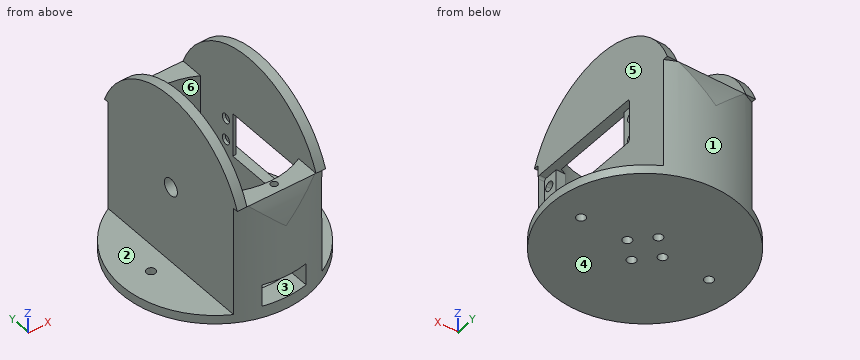
Autodesk Inventor part; units mm, degrees
ref_plane "РабПлоскость2" through (0, -42.5, 39) normal (0, -1, 0) x (1, 0, 0)
ref_plane "YZ Plane" through (0, 0, 0) normal (1, 0, 0) x (0, 1, 0)
ref_plane "XZ Plane" through (0, 0, 0) normal (0, 1, 0) x (-1, 0, 0)
sketch "Эскиз1" plane through (0, 0, 0) normal (0, 0, 1) x (1, 0, 0)
  circle A0 centre (29, 0) radius 2
  circle A1 centre (-29, 0) radius 2
  circle A2 centre (0, 8) radius 2
  circle A3 centre (8, 0) radius 2
  circle A4 centre (0, -8) radius 2
  circle A5 centre (-8, 0) radius 2
  circle A6 centre (0, 0) radius 42.5
  circle A7 centre (29, 0) radius 2
  circle A8 centre (-29, 0) radius 2
  circle A9 centre (0, 8) radius 2
  circle A10 centre (8, 0) radius 2
  circle A11 centre (0, -8) radius 2
  circle A12 centre (-8, 0) radius 2
  circle A13 centre (0, 0) radius 42.5
extrude "Выдавливание1" add sketch "Эскиз1" along normal blind 4
sketch "Эскиз16" plane through (0, 0, 4) normal (0, 0, 1) x (1, 0, 0)
  line L0 (-20, -37.5) -> (-20, 37.5)
  line L1 (20, 37.5) -> (20, -37.5)
  line L2 (20, -42.5) -> (-20, 42.5) construction
  line L3 (-20, -42.5) -> (20, 42.5) construction
  circle A0 centre (0, 0) radius 42.5
  arc A1 (-20, -37.5) -> (20, -37.5) centre (0, 0) ccw
  arc A2 (20, 37.5) -> (-20, 37.5) centre (0, 0) ccw
extrude "Выдавливание14" add sketch "Эскиз16" along normal blind 50 contours L0 A0 L1
sketch "Эскиз17" plane through (0, 0, 54) normal (0, 0, 1) x (1, 0, 0)
  line L0 (-15.66, -29.3625) -> (-15.66, 29.3625)
  line L1 (15.66, 29.3625) -> (15.66, -29.3625)
  line L2 (15.66, -33.2775) -> (-15.66, 33.2775) construction
  line L3 (-15.66, -33.2775) -> (15.66, 33.2775) construction
  arc A0 (-15.66, -29.3625) -> (15.66, -29.3625) centre (0, 0) ccw
  arc A1 (15.66, 29.3625) -> (-15.66, 29.3625) centre (0, 0) ccw
  arc A2 (-15.66, -29.3625) -> (15.66, -29.3625) centre (0, 0) ccw
  arc A3 (15.66, 29.3625) -> (-15.66, 29.3625) centre (0, 0) ccw
extrude "Выдавливание15" cut sketch "Эскиз17" against normal up to surface (50 mm away)
sketch "Эскиз23" plane through (-20, -37.5, 4) normal (-1, 0, 0) x (0, 0, 1)
  line L0 (0, 39.5) -> (0, 35.5)
  line L1 (0, 37.5) -> (35, 37.5)
  circle A0 centre (35, 37.5) radius 3.9
  point P0 (-4, 37.5)
  dimension "d73" = 35
  dimension "d74" = 7.8
extrude "Выдавливание21" cut sketch "Эскиз23" against normal blind 54
sketch "Эскиз26" plane through (20, -37.5, 4) normal (1, 0, 0) x (0, 0, -1)
  circle A0 centre (-35, 37.5) radius 3.9
  line L0 (-45, 47.5) -> (-25, 47.5)
  line L1 (-25, 47.5) -> (-25, 53.5)
  arc A1 (-25, 53.5) -> (-26, 54.5) centre (-26, 53.5) ccw
  line L2 (-26, 54.5) -> (-28.85, 54.5)
  line L3 (-28.85, 54.5) -> (-28.85, 53.434)
  arc A2 (-31.25, 53.434) -> (-28.85, 53.434) centre (-30.05, 51.65) ccw
  line L4 (-31.25, 53.434) -> (-31.25, 54.5)
  line L5 (-31.25, 54.5) -> (-38.75, 54.5)
  line L6 (-38.75, 54.5) -> (-38.75, 53.434)
  arc A3 (-41.15, 53.434) -> (-38.75, 53.434) centre (-39.95, 51.65) ccw
  line L7 (-41.15, 53.434) -> (-41.15, 54.5)
  line L8 (-41.15, 54.5) -> (-44, 54.5)
  arc A4 (-44, 54.5) -> (-45, 53.5) centre (-44, 53.5) ccw
  line L9 (-45, 53.5) -> (-45, 47.5)
  line L10 (-38.75, -0.2) -> (-38.75, 0.866)
  line L11 (-31.25, -0.2) -> (-38.75, -0.2)
  line L12 (-31.25, 0.866) -> (-31.25, -0.2)
  arc A5 (-28.85, 0.866) -> (-31.25, 0.866) centre (-30.05, 2.65) ccw
  line L13 (-28.85, -0.2) -> (-28.85, 0.866)
  line L14 (-26, -0.2) -> (-28.85, -0.2)
  arc A6 (-26, -0.2) -> (-25, 0.8) centre (-26, 0.8) ccw
  line L15 (-25, 6.8) -> (-25, 0.8)
  line L16 (-45, 6.8) -> (-25, 6.8)
  line L17 (-45, 0.8) -> (-45, 6.8)
  arc A7 (-45, 0.8) -> (-44, -0.2) centre (-44, 0.8) ccw
  line L18 (-41.15, -0.2) -> (-44, -0.2)
  line L19 (-41.15, 0.866) -> (-41.15, -0.2)
  arc A8 (-38.75, 0.866) -> (-41.15, 0.866) centre (-39.95, 2.65) ccw
  line L20 (-25, 47.5) -> (-25, 6.8)
  line L21 (-45, 6.8) -> (-45, 47.5)
  line L22 (-45, 47.5) -> (-25, 47.5)
  circle A9 centre (-35, 37.5) radius 1.25
  circle A10 centre (-35, 37.5) radius 3.4957
  circle A11 centre (-35, 37.5) radius 2.6787
  circle A12 centre (-35, 37.5) radius 5.4
  line L23 (-28.85, -0.2) -> (-31.25, -0.2)
  line L24 (-38.75, -0.2) -> (-41.15, -0.2)
  line L25 (-31.25, -0.2) -> (-34.5, -0.2)
  line L26 (-31.25, 54.5) -> (-38.75, 54.5)
  line L27 (-28.85, 54.5) -> (-31.25, 54.5)
  line L28 (-31.25, 54.5) -> (-38.75, 54.5)
  line L29 (-38.75, 54.5) -> (-41.15, 54.5)
  circle A13 centre (-30.05, 51.65) radius 2.15
  circle A14 centre (-39.95, 51.65) radius 2.15
  arc A15 (-38.75, 0.866) -> (-41.15, 0.866) centre (-39.95, 2.65) ccw
  circle A16 centre (-39.95, 2.65) radius 2.15
  circle A17 centre (-30.05, 2.65) radius 2.15
  circle A18 centre (-35, 37.5) radius 42.5
  line L30 (4, 80) -> (-50, 80)
  line L31 (-50, 0) -> (-50, -5)
  line L32 (-50, -2.2649) -> (-50, -5)
  line L33 (4, -5) -> (-50, -5)
  line L34 (-35, -5) -> (-50, -5)
  line L35 (4, -5) -> (-50, -5)
  line L36 (-50, 80) -> (-50, 75)
  line L37 (-50, 77.2649) -> (-50, 80)
  line L38 (-50, 80) -> (-35, 80)
  line L39 (4, 80) -> (-50, 80)
  point P0 (4, 37.5)
  point P1 (-45, 27.15)
extrude "Выдавливание23" cut sketch "Эскиз26" against normal blind 10 contours A0 | L0 L20 L16 L21 | A9 | A10 | A11 | A12
sketch "Эскиз27" plane through (20, -37.5, 4) normal (1, 0, 0) x (0, 0, -1)
  circle A0 centre (-35, 37.5) radius 3.9
  line L0 (-45, 47.5) -> (-25, 47.5)
  line L1 (-25, 47.5) -> (-25, 53.5)
  arc A1 (-25, 53.5) -> (-26, 54.5) centre (-26, 53.5) ccw
  line L2 (-26, 54.5) -> (-28.85, 54.5)
  line L3 (-28.85, 54.5) -> (-28.85, 53.434)
  arc A2 (-31.25, 53.434) -> (-28.85, 53.434) centre (-30.05, 51.65) ccw
  line L4 (-31.25, 53.434) -> (-31.25, 54.5)
  line L5 (-31.25, 54.5) -> (-38.75, 54.5)
  line L6 (-38.75, 54.5) -> (-38.75, 53.434)
  arc A3 (-41.15, 53.434) -> (-38.75, 53.434) centre (-39.95, 51.65) ccw
  line L7 (-41.15, 53.434) -> (-41.15, 54.5)
  line L8 (-41.15, 54.5) -> (-44, 54.5)
  arc A4 (-44, 54.5) -> (-45, 53.5) centre (-44, 53.5) ccw
  line L9 (-45, 53.5) -> (-45, 47.5)
  line L10 (-38.75, -0.2) -> (-38.75, 0.866)
  line L11 (-31.25, -0.2) -> (-38.75, -0.2)
  line L12 (-31.25, 0.866) -> (-31.25, -0.2)
  arc A5 (-28.85, 0.866) -> (-31.25, 0.866) centre (-30.05, 2.65) ccw
  line L13 (-28.85, -0.2) -> (-28.85, 0.866)
  line L14 (-26, -0.2) -> (-28.85, -0.2)
  arc A6 (-26, -0.2) -> (-25, 0.8) centre (-26, 0.8) ccw
  line L15 (-25, 6.8) -> (-25, 0.8)
  line L16 (-45, 6.8) -> (-25, 6.8)
  line L17 (-45, 0.8) -> (-45, 6.8)
  arc A7 (-45, 0.8) -> (-44, -0.2) centre (-44, 0.8) ccw
  line L18 (-41.15, -0.2) -> (-44, -0.2)
  line L19 (-41.15, 0.866) -> (-41.15, -0.2)
  arc A8 (-38.75, 0.866) -> (-41.15, 0.866) centre (-39.95, 2.65) ccw
  line L20 (-25, 47.5) -> (-25, 6.8)
  line L21 (-45, 6.8) -> (-45, 47.5)
  line L22 (-45, 47.5) -> (-25, 47.5)
  circle A9 centre (-35, 37.5) radius 1.25
  circle A10 centre (-35, 37.5) radius 3.4957
  circle A11 centre (-35, 37.5) radius 2.6787
  circle A12 centre (-35, 37.5) radius 5.4
  line L23 (-28.85, -0.2) -> (-31.25, -0.2)
  line L24 (-38.75, -0.2) -> (-41.15, -0.2)
  line L25 (-31.25, -0.2) -> (-34.5, -0.2)
  line L26 (-31.25, 54.5) -> (-38.75, 54.5)
  line L27 (-28.85, 54.5) -> (-31.25, 54.5)
  line L28 (-31.25, 54.5) -> (-38.75, 54.5)
  line L29 (-38.75, 54.5) -> (-41.15, 54.5)
  circle A13 centre (-30.05, 51.65) radius 2.15
  circle A14 centre (-39.95, 51.65) radius 2.15
  arc A15 (-38.75, 0.866) -> (-41.15, 0.866) centre (-39.95, 2.65) ccw
  circle A16 centre (-39.95, 2.65) radius 2.15
  circle A17 centre (-30.05, 2.65) radius 2.15
  point P0 (4, 37.5)
  point P1 (4, 37.5)
  point P2 (-45, 27.15)
extrude "Выдавливание24" cut sketch "Эскиз27" against normal blind 3 contours L9 A4 L8 L7 A3 L6 L5 L4 A2 L3 L2 A1 L1 L0 | L16 L15 A6 L14 L13 A5 L12 L11 L10 A8 L19 L18 A7 L17 | L29 L6 A14 L7 | L3 A13 L4 L27 | A14 A3 | L19 A16 L10 L24 | A2 A13 | L23 L12 A17 L13 | A8 A16 | A17 A5
sketch "Эскиз28" plane through (17, -37.5, 4) normal (1, 0, 0) x (0, 0, -1)
  circle A0 centre (-35, 37.5) radius 3.9
  line L0 (-45, 47.5) -> (-25, 47.5)
  line L1 (-25, 47.5) -> (-25, 53.5)
  arc A1 (-25, 53.5) -> (-26, 54.5) centre (-26, 53.5) ccw
  line L2 (-26, 54.5) -> (-28.85, 54.5)
  line L3 (-28.85, 54.5) -> (-28.85, 53.434)
  arc A2 (-31.25, 53.434) -> (-28.85, 53.434) centre (-30.05, 51.65) ccw
  line L4 (-31.25, 53.434) -> (-31.25, 54.5)
  line L5 (-31.25, 54.5) -> (-38.75, 54.5)
  line L6 (-38.75, 54.5) -> (-38.75, 53.434)
  arc A3 (-41.15, 53.434) -> (-38.75, 53.434) centre (-39.95, 51.65) ccw
  line L7 (-41.15, 53.434) -> (-41.15, 54.5)
  line L8 (-41.15, 54.5) -> (-44, 54.5)
  arc A4 (-44, 54.5) -> (-45, 53.5) centre (-44, 53.5) ccw
  line L9 (-45, 53.5) -> (-45, 47.5)
  line L10 (-38.75, -0.2) -> (-38.75, 0.866)
  line L11 (-31.25, -0.2) -> (-38.75, -0.2)
  line L12 (-31.25, 0.866) -> (-31.25, -0.2)
  arc A5 (-28.85, 0.866) -> (-31.25, 0.866) centre (-30.05, 2.65) ccw
  line L13 (-28.85, -0.2) -> (-28.85, 0.866)
  line L14 (-26, -0.2) -> (-28.85, -0.2)
  arc A6 (-26, -0.2) -> (-25, 0.8) centre (-26, 0.8) ccw
  line L15 (-25, 6.8) -> (-25, 0.8)
  line L16 (-45, 6.8) -> (-25, 6.8)
  line L17 (-45, 0.8) -> (-45, 6.8)
  arc A7 (-45, 0.8) -> (-44, -0.2) centre (-44, 0.8) ccw
  line L18 (-41.15, -0.2) -> (-44, -0.2)
  line L19 (-41.15, 0.866) -> (-41.15, -0.2)
  arc A8 (-38.75, 0.866) -> (-41.15, 0.866) centre (-39.95, 2.65) ccw
  line L20 (-25, 47.5) -> (-25, 6.8)
  line L21 (-45, 6.8) -> (-45, 47.5)
  line L22 (-45, 47.5) -> (-25, 47.5)
  circle A9 centre (-35, 37.5) radius 1.25
  circle A10 centre (-35, 37.5) radius 3.4957
  circle A11 centre (-35, 37.5) radius 2.6787
  circle A12 centre (-35, 37.5) radius 5.4
  line L23 (-28.85, -0.2) -> (-31.25, -0.2)
  line L24 (-38.75, -0.2) -> (-41.15, -0.2)
  line L25 (-31.25, -0.2) -> (-34.5, -0.2)
  line L26 (-31.25, 54.5) -> (-38.75, 54.5)
  line L27 (-28.85, 54.5) -> (-31.25, 54.5)
  line L28 (-31.25, 54.5) -> (-38.75, 54.5)
  line L29 (-38.75, 54.5) -> (-41.15, 54.5)
  circle A13 centre (-30.05, 51.65) radius 2.15
  circle A14 centre (-39.95, 51.65) radius 2.15
  arc A15 (-38.75, 0.866) -> (-41.15, 0.866) centre (-39.95, 2.65) ccw
  circle A16 centre (-39.95, 2.65) radius 2.15
  circle A17 centre (-30.05, 2.65) radius 2.15
  point P0 (4, 37.5)
  point P1 (4, 37.5)
  point P2 (-45, 27.15)
extrude "Выдавливание25" cut sketch "Эскиз28" against normal blind 15 contours A14 A3 | A2 A13 | A8 A16 | A17 A5
sketch "Эскиз29" plane through (20, -37.5, 4) normal (1, 0, 0) x (0, 0, -1)
  circle A0 centre (-35, 37.5) radius 3.9
  circle A1 centre (-35, 37.5) radius 42.5
  line L0 (4, 80) -> (-50, 80)
  line L1 (-50, -2.2649) -> (-50, -5)
  line L2 (-50, -5) -> (-35, -5)
  line L3 (4, -5) -> (-50, -5)
  line L4 (-50, 80) -> (-50, 75)
  line L5 (-50, 77.2649) -> (-50, 80)
  line L6 (-50, 80) -> (-35, 80)
  point P0 (4, 37.5)
extrude "Выдавливание26" cut sketch "Эскиз29" against normal blind 46.75 contours A1 L4 L0 | L2 L1 A1
sketch "Эскиз30" plane through (20, -37.5, 4) normal (1, 0, 0) x (0, 0, -1)
  circle A0 centre (-35, 37.5) radius 3.9
  circle A1 centre (-35, 37.5) radius 42.5
  line L0 (-50, 0) -> (-50, -2.2649)
  line L1 (-50, -2.2649) -> (-50, 77.2649)
  line L2 (-50, 8.1375) -> (-50, 66.8625)
  point P0 (4, 37.5)
extrude "Выдавливание27" add sketch "Эскиз30" against normal up to surface (4.34 mm away) contours L1 L0 A1 picked at (-59.1667, 37.5)
sketch "Эскиз31" plane through (-20, -37.5, 4) normal (-1, 0, 0) x (0, 0, 1)
  circle A0 centre (35, 37.5) radius 3.9
  circle A1 centre (35, 37.5) radius 42.5
  line L0 (50, 75) -> (50, 77.2649)
  line L1 (50, 77.2649) -> (50, -2.2649)
  line L2 (50, 66.8625) -> (50, 8.1375)
  circle A2 centre (35, 37.5) radius 3.9
  point P0 (-4, 37.5)
  point P1 (-4, 37.5)
extrude "Выдавливание28" add sketch "Эскиз31" against normal up to surface (4.34 mm away) contours A1 L1 L0 picked at (59.1667, 37.5)
sketch "Эскиз32" plane through (-20, -37.5, 4) normal (-1, 0, 0) x (0, 0, 1)
  circle A0 centre (35, 37.5) radius 3.9
  line L0 (0, 0) -> (0, 75)
  line L1 (0, 0) -> (50, 0)
  line L2 (50, 0) -> (50, -2.2649)
  arc A1 (50, -2.2649) -> (50, 77.2649) centre (35, 37.5) ccw
  line L3 (50, 77.2649) -> (50, 75)
  line L4 (0, 75) -> (50, 75)
  point P0 (-4, 37.5)
ref_plane "РабПлоскость2" through (0, -42.5, 39) normal (0, -1, 0) x (1, 0, 0)
sketch "Эскиз33" plane through (0, -42.5, 39) normal (0, -1, 0) x (1, 0, 0)
  line L0 (-10, -33.6111) -> (10, -33.6111)
  line L1 (10, -33.6111) -> (10, -23.6111)
  line L2 (10, -23.6111) -> (-10, -23.6111)
  line L3 (-10, -23.6111) -> (-10, -33.6111)
  line L4 (-10, -33.6111) -> (10, -23.6111) construction
  line L5 (10, -33.6111) -> (-10, -23.6111) construction
  point P0 (0, -39)
  point P1 (0, -28.6111)
  dimension "d92" = 20
  dimension "d93" = 10
extrude "Выдавливание29" cut sketch "Эскиз33" against normal blind 18.75
sketch "Эскиз34" plane through (0, 0, 54) normal (0, 0, 1) x (1, 0, 0)
  line L0 (0, 0) -> (0, -35.407)
  circle A0 centre (0, -35.407) radius 1.5
  dimension "d96" = 35.407
  dimension "d97" = 3
extrude "Выдавливание30" cut sketch "Эскиз34" against normal blind 5
pattern_circular "Круговой массив1" count 2 over 360 about axis through (0, 0, 0) along (0, 0, 1) of "Выдавливание30"
properties part number "joint3_main" material "Пластик АБС"
The listing builds one solid part. Answer for the finished solid, in the listing's coordinates (mm). Face numbers are marked on the shaded views. A direction names the side the tool comes from. Coordinates: 2 decimals unless noted, no trailing zeros. Write each loop counter-clockwise with the first axis right and the second up, starting at its lowest first coordinate (ties: lowest second). Pieces come first, ordered by that corner, then holes. Notation, with made-up numbers: (51, 76.25) - (81, 76.25) arc R7 ccw to (81, 81.25) - close; hole circle Ø4 at (52, 8). An arc over 180 degrees is marked (long way). One line per item, written item: value.
1) Consider line 1 along Y through (x, z) = (0, 2); line 2 along X through (y, z) = (19, 73); line 3 along Z through (x, y) = (11.5, -34.85). Determine where each line is inside the solid, lowest interval first. Write a range as from..to.
Geometry check:
line 1: y = -42.5..-10, -6..6, 10..42.5
line 2: x = -20..-15.66, 15.66..20
line 3: z = 0..31.9, 36.2..41.8, 46.1..54
2) For a pull along X with two mould halves and no side action, classify the marked faces 4, 5 and 6 as pulls with the +X half, pulls with the -X half, needs draft (parallel to the pull), parting line crosses it, or undercut.
Geometry check:
face 4: needs draft
face 5: pulls with the +X half
face 6: undercut
3) Each of these flat-tipped pins is pushed along its axis until it touches: pin 1 Ø10 at (x, z) = (-10.5, 49) entering from +Y; pin 2 Ø8 at (y, z) = (21.5, 40) entering from +X; pin 3 Ø5 at (y, z) = (-35, 8.5) entering from -X; pin 4 Ø8.5 at (x, y) = (4, -34.5) entering from -Z. Where does it stop, or does it pass through?
Geometry check:
pin 1: stops at y = 41.96
pin 2: stops at x = 20
pin 3: stops at x = -20
pin 4: stops at z = 0
4) Find section A-A (z = 73.5). Give the vertices of the cut face in (x, y).
Geometry check:
outline: (-20, -24.82) - (-15.66, -24.82) - (-15.66, 24.82) - (-20, 24.82) - close; (15.66, -24.82) - (20, -24.82) - (20, 24.82) - (15.66, 24.82) - close
5) Find section B-B (x = 29). Give the vertices of the cut face in (y, z), and give its area (3 significant figures).
Geometry check:
outline: (-31.07, 0) - (-2, 0) - (-2, 4) - (-31.07, 4) - close; (2, 0) - (31.07, 0) - (31.07, 4) - (2, 4) - close
area: 233 mm2
6) Find section C-C (y = 0). Count the separate pieces of the cut face and the enclosed holes in it, and give its area (3 significant figures).
Geometry check:
separate pieces: 7
enclosed holes: 0
area: 828 mm2
7) A tool of negligible diameter and unlimited length cuts with its end or side. For the marked faces 1, 2 and 3, from which of +Z, -Z, +X, -X, +Y, -Y can it reach the whole face along a straight path? Write none if from no direction.
Geometry check:
face 1: -Z
face 2: +Z, -X, +Y, -Y
face 3: -Y
